from build123d import *

# Parameters (mm, degrees)
BOSS_EXTRUDE1_DEPTH     = 6.35
CAVITY1_START           = -13.966782317
CAVITY1_OUTLINE_R       = 12.7
CAVITY1_DEPTH           = 20.041848041
CUT_EXTRUDE2_REACH      = 287.468
CUT_EXTRUDE2_END_RADIUS = 12.7
SKETCH6_W               = 25.4
SKETCH6_H               = 12.7


# Read off the part's stored shape, not the designer's step: Cavity1
with BuildPart() as part:
    # Sketch1 → Boss-Extrude1 (new, symmetric)
    with BuildSketch(Plane(origin=(0, 0, 0), x_dir=(1, 0, 0), z_dir=(0, 1, 0))):
        Polygon((-215.9, 76.2), (215.9, 76.2), (241.3, 76.2), (241.3, 0), (215.9, 0), (215.9, -76.2), (-215.9, -76.2), (-215.9, 0), (-241.3, 0), (-241.3, 76.2), align=None)
    extrude(amount=BOSS_EXTRUDE1_DEPTH, both=True)

    # Cavity1 outline → Cavity1 (cut)
    with BuildSketch(Plane(origin=(0, 0, 0), x_dir=(1, 0, 0), z_dir=(0, 0.9651827234760059, -0.261576585923588)).offset(CAVITY1_START)):
        with Locations((-50.8, -14.559690973)):
            Circle(CAVITY1_OUTLINE_R)
    extrude(amount=CAVITY1_DEPTH, mode=Mode.SUBTRACT)

    # Cut-Extrude2: up to this cylinder (the profile starts outside it)
    cut_extrude2_end = Plane(origin=(-50.8, -15.429678905, 19.266542232), z_dir=(0, 0.965182723476006, -0.2615765859235875)) * Cylinder(CUT_EXTRUDE2_END_RADIUS, 601.336, mode=Mode.PRIVATE)
    # Sketch6 → Cut-Extrude2 (cut, up to the surface)
    with BuildSketch(Plane.XY.offset(76.2), mode=Mode.PRIVATE) as cut_extrude2_sk1:
        with Locations((-50.8, 0)):
            Rectangle(SKETCH6_W, SKETCH6_H)
    cut_extrude2_tool1 = extrude(cut_extrude2_sk1.sketch, amount=-CUT_EXTRUDE2_REACH, mode=Mode.PRIVATE) - cut_extrude2_end
    add(cut_extrude2_tool1.solids().sort_by_distance((-50.8, 0, 76.2))[0], mode=Mode.SUBTRACT)


solid = part.part
Read the model definition and answer for the solid it produces. Units are mm, in the model's axes. A direction names the side the tool comes from. Coordinates: 2 decimals unless noted, no trailing zeros. Loops run counter-clockwise (first coordinate to the right, second up) from the corner with the lowest first, then second, coordinate; pieces in that order, holes last.
Q1. Each of these flat-tipped pins is pushed along its axis until it touches: pin 1 Ø6.5 at (y, z) = (-3, 32.5) entering from +X; pin 2 Ø6.5 at (x, y) = (228, 0) entering from +Z. Where does it stop, or does it pass through?
Q2. The part is cut by section A-A on z = 52. Write down the section's boundary in (x, y).
Q3. The part is cut by section B-B on x = -59. Write down the section's boundary in (y, z).
Q4. Which of the six approach directions +Z, -Z, +X, -X, +Y, -Y give full straight-line access (tool end or side, diameter ignored) to faces 1 (the face through (-228, 0, 0)), 2 (the face through (3, 0, -76.2)), 3 (the face through (215.9, 0, 38)), 4 (the face through (3, -6.35, -1)), 5 (the face through (-63.5, 0, 45))?
Q5. Consider probe 1 along X at (y, z) = (2, 65.5); probe 2 along Z at (x, y) = (-217, -4.75); probe 3 along Z at (x, y) = (-48, -5). Determine where each line is inside the solid, lowest interval first.
Results below:
1. pin 1: stops at x = 215.9
1. pin 2: stops at z = 0
2. outline: (-215.9, -6.35) - (-63.5, -6.35) - (-63.5, 6.35) - (-215.9, 6.35) - close; (-38.1, -6.35) - (215.9, -6.35) - (215.9, 6.35) - (-38.1, 6.35) - close
3. outline: (-6.35, -76.2) - (6.35, -76.2) - (6.35, 3.32) - (-6.35, 6.76) - close
4. face 1: +Z, -X, +Y, -Y
4. face 2: -Z, +X, -X, +Y, -Y
4. face 3: +Z, +X, +Y, -Y
4. face 4: +Z, -Z, +X, -X, -Y
4. face 5: +Z, +Y, -Y
5. probe 1: x = -215.9 to -63.5, -38.1 to 215.9
5. probe 2: z = -76.2 to 0
5. probe 3: z = -76.2 to 3.61
